Check sheet for the drawn part. Datum: minimum x, y, z corner. Units: mm. A direction names the side the tool comes from. Coordinates: 2 decimals unless noted, no trailing zeros. Loops run counter-clockwise (first coordinate to the right, second up) from the corner with the lowest first, then second, coordinate; pieces in that order, holes last. Notation, with made-up numbers: (-7.5, 40) - (26.5, 40) arc R19 cw to (26.5, 62) - close; hole circle Ø8 at (37, 87). An arc over 180 degrees is marked (long way). Write item = value, one per line. Start each with the question number.
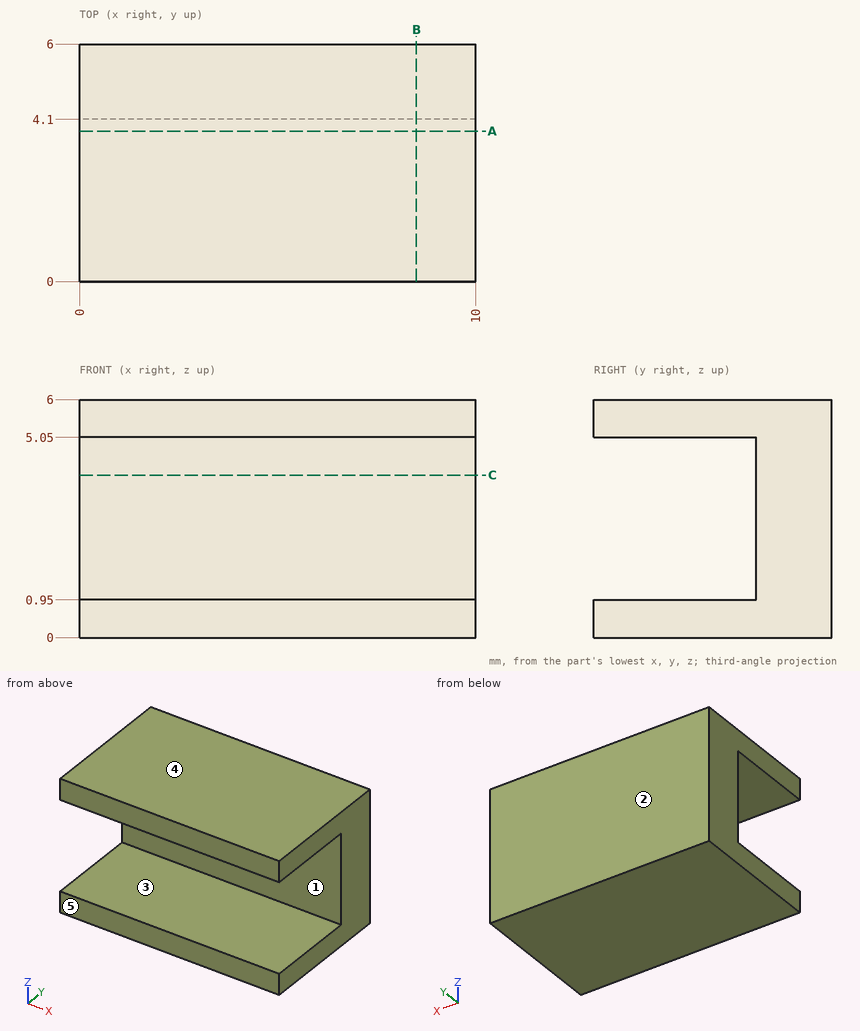
(1) Depth check by flat-ended pin: pin 1 (1.5 mm diameter, centred on x = 4.5, z = 3, fed in from -Y); pin 2 (2 mm diameter, centred on y = 2, z = 2, fed in from +X). Enter the tip coordinate at first touch or a pass-through.
(2) Draft check along Z on the marked faces 3, 4 and 5. Enter one of: pulls with the +Z half, pulls with the -Z half, needs draft (parallel to the pull), parting line crosses it, or undercut.
(3) Sectioned sample at B-B on x = 8.5. Enter the section's corners in (y, z).
(4) Sectioned sample at A-A on y = 3.8. Enter the section's corners in (x, z).
(5) Tool access check on the marked faces 1 and 2. Record the directions out of +Z, -Z, +X, -X, +Y, -Y that give a thin tool (end or side, any length) a straight path to the whole face; none if there is none.
(6) Sectioned sample at C-C on z = 4.1. Enter the section's corners in (x, y), plus the area to 3 significant figures.
(7) Scan lines: line 1 (Z direction, x = 2.75, y = 2.35); line 2 (Y direction, x = 0.5, z = 2.9). Record each from-to range of solid material in increasing order.
Working result:
q1.pin_1 = 4.1
q1.pin_2 = through
q2.face_3 = undercut
q2.face_4 = pulls with the +Z half
q2.face_5 = needs draft
q3.outline = (0, 0) - (6, 0) - (6, 6) - (0, 6) - (0, 5.05) - (4.1, 5.05) - (4.1, 0.95) - (0, 0.95) - close
q4.outline = (0, 0) - (10, 0) - (10, 0.95) - (0, 0.95) - close; (0, 5.05) - (10, 5.05) - (10, 6) - (0, 6) - close
q5.face_1 = +X, -X, -Y
q5.face_2 = +Z, -Z, +X, -X, +Y
q6.outline = (0, 4.1) - (10, 4.1) - (10, 6) - (0, 6) - close
q6.area = 19.0 mm2
q7.line_1 = 0 to 0.95, 5.05 to 6
q7.line_2 = 4.1 to 6
